Verification items for the finished model (mm, model axes). Face numbers are marked on the shaded views. A direction names the side the tool comes from. Coordinates: 2 decimals unless noted, no trailing zeros. Order: outer loops, then holes, each group sorted by start corner. A loop starts at its lowest first (then second) coordinate and runs counter-clockwise, first axis right, second up. Notation, with made-up numbers: M 39.25,-33 L 85.25,-33 A26 ccw 85.25,-16 Z; hole C -9,-19.5 d10. An arc over 180 degrees is marked long. Return JSON: item names as keys, results as strings.
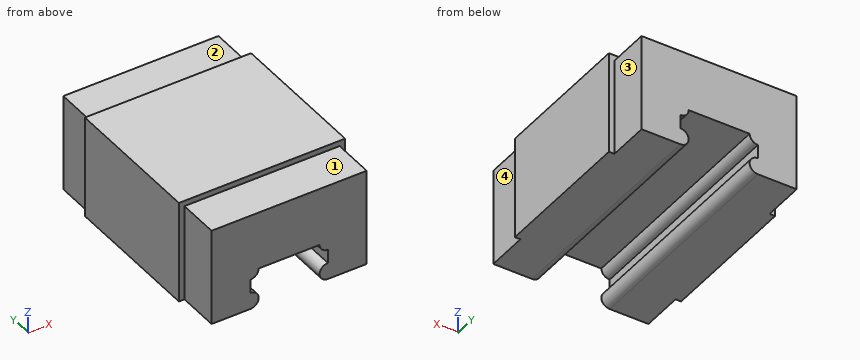
```python
from build123d import *

# Parameters (mm, degrees)
F1_DEPTH = 82
F2_W     = 60
F2_H     = 15
F3_DEPTH = 2
F4_W     = 2
F4_H     = 15
F5_DEPTH = 35


with BuildPart() as f1:
    # F0 (on Front) → F1 (new body)
    with BuildSketch(Plane.XZ):
        with BuildLine():
            ThreePointArc((16, 11), (18.12132, 11.87868), (19, 14))
            Line((19, 14), (41, 14))
            ThreePointArc((41, 14), (41.87868, 11.87868), (44, 11))
            Line((44, 11), (44, 6))
            ThreePointArc((44, 6), (41, 3), (44, 0))
            Line((44, 0), (60, 0))
            Line((60, 0), (60, 37))
            Line((60, 37), (0, 37))
            Line((0, 37), (0, 0))
            Line((0, 0), (16, 0))
            ThreePointArc((16, 0), (19, 3), (16, 6))
            Line((16, 6), (16, 11))
        make_face()
    extrude(amount=F1_DEPTH)

    # F2 (on face) → F3 (cut)
    with BuildSketch(Plane.XY.offset(37)):
        with Locations((30, -7.5)):
            Rectangle(F2_W, F2_H)
        with Locations((30, -74.5)):
            Rectangle(F2_W, F2_H)
    extrude(amount=-F3_DEPTH, mode=Mode.SUBTRACT)

    # F4 (on face) → F5 (cut)
    with BuildSketch(Plane.XY.offset(35)):
        with Locations((1, -7.5)):
            Rectangle(F4_W, F4_H)
        with Locations((59, -7.5)):
            Rectangle(F4_W, F4_H)
        with Locations((1, -74.5)):
            Rectangle(F4_W, F4_H)
        with Locations((59, -74.5)):
            Rectangle(F4_W, F4_H)
    extrude(amount=-F5_DEPTH, mode=Mode.SUBTRACT)


solid = f1.part
```
Q1. Cross-section at B-B, the plane x = 4.5. Record the boundary of the cut face in (y, z).
Values:
{"outline": "M -82,0 L 0,0 L 0,35 L -15,35 L -15,37 L -67,37 L -67,35 L -82,35 Z"}
Q2. Cross-section at A-A, the plane z = 7. Record the boundary of the cut face in (x, y).
Values:
{"outline": "M 0,-67 L 2,-67 L 2,-82 L 16,-82 L 16,0 L 2,0 L 2,-15 L 0,-15 Z; M 44,-82 L 58,-82 L 58,-67 L 60,-67 L 60,-15 L 58,-15 L 58,0 L 44,0 Z"}
Q3. Tool access check on the marked faces 1, 2, 3 and 4. Record the directions out of +Z, -Z, +X, -X, +Y, -Y that give a thin tool (end or side, any length) a straight path to the whole face; none if there is none.
Values:
{"face 1": "+Z, +X, -X, -Y", "face 2": "+Z, +X, -X, +Y", "face 3": "+Z, -Z, +X, +Y", "face 4": "+Z, -Z, +X, -Y"}
Q4. Material ranges on line 1 along X through (y, z) = (-75, 6.5); line 2 along X through (y, z) = (-58, 7); line 3 along X through (y, z) = (-5.5, 26), recorded low to high.
Values:
{"line 1": "2 to 16, 44 to 58", "line 2": "0 to 16, 44 to 60", "line 3": "2 to 58"}
Q5. Cross-section at D-D, the plane z = 3. Record the boundary of the cut face in (x, y).
Values:
{"outline": "M 0,-67 L 2,-67 L 2,-82 L 19,-82 L 19,0 L 2,0 L 2,-15 L 0,-15 Z; M 41,-82 L 58,-82 L 58,-67 L 60,-67 L 60,-15 L 58,-15 L 58,0 L 41,0 Z"}
Q6. Cross-section at C-C, the plane y = -60. Record the boundary of the cut face in (x, z).
Values:
{"outline": "M 0,0 L 16,0 A3 ccw 16,6 L 16,11 A3 ccw 19,14 L 41,14 A3 ccw 44,11 L 44,6 A3 ccw 44,0 L 60,0 L 60,37 L 0,37 Z"}
Q7. Go/stop test with flat-tipped pins: pin 1 (4.5 mm diameter, centred on x = 21.5, y = -11, fed in from +Z); pin 2 (4.5 mm diameter, centred on y = -72, z = 20, fed in from -X); pin 3 (17.5 mm diameter, centred on x = 35, y = -25, fed in from -Z). Record where each tip stops, or that it passes through.
Values:
{"pin 1": "z = 35", "pin 2": "x = 2", "pin 3": "z = 0.01"}
